from build123d import *
from build123d.topology import SkipClean

# Parameters (mm, degrees)
BOSS_EXTRUDE1_DEPTH   = 0.00254
BOSS_EXTRUDE1_2_DEPTH = 0.00254
BOSS_EXTRUDE1_3_DEPTH = 0.00254
BOSS_EXTRUDE1_4_DEPTH = 0.00254
SKETCH1_3_R           = 4.7625
BOSS_EXTRUDE2_DEPTH   = 1.9812
SKETCH1_6_R           = 14.02334
BOSS_EXTRUDE4_DEPTH   = 1.9812
SKETCH1_7_R           = 18.669
SKETCH1_7_R_2         = 14.02334
BOSS_EXTRUDE5_DEPTH   = 21.4122
BOSS_EXTRUDE6_DEPTH   = 21.4122
BOSS_EXTRUDE7_DEPTH   = 80.264
SKETCH9_R             = 4.064
CUT_EXTRUDE6_DEPTH    = 11.938
SKETCH10_R            = 3.556
CUT_EXTRUDE7_DEPTH    = 25.4


with BuildPart() as part:
    # Sketch1 → Boss-Extrude1 (new body)
    with BuildSketch(Plane.XY):
        with BuildLine():
            add(Edge.make_bspline(
                [(-11.267882352, 10.780839024), (-10.870534927, 8.031966006), (-8.087704817, 8.031966006), (-5.304874707, 8.031966006), (-4.907527282, 10.780839024)],
                knots=[3.284867705, 3.284867705, 3.284867705, 4.71238898, 4.71238898, 6.139910255, 6.139910255, 6.139910255], degree=2, weights=[1, 0.755905209, 1, 0.755905209, 1]))
            add(Edge.make_bspline(
                [(-4.907527282, 10.780839024), (-4.377808345, 14.445466006), (-8.087704817, 14.445466006), (-11.79760129, 14.445466006), (-11.267882352, 10.780839024)],
                knots=[6.139910255, 6.139910255, 6.139910255, 7.853981634, 7.853981634, 9.568053013, 9.568053013, 9.568053013], degree=2, weights=[1, 0.654681079, 1, 0.654681079, 1]))
        make_face()
    extrude(amount=BOSS_EXTRUDE1_DEPTH)



with BuildPart() as body_2:
    # Sketch1 → Boss-Extrude1 2 (new body)
    with BuildSketch(Plane.XY):
        with BuildLine():
            add(Edge.make_bspline(
                [(-15.980077835, -0.291711529), (-13.231204817, 0.105635896), (-13.231204817, 2.888466006), (-13.231204817, 5.671296116), (-15.980077835, 6.068643541)],
                knots=[3.284867705, 3.284867705, 3.284867705, 4.71238898, 4.71238898, 6.139910255, 6.139910255, 6.139910255], degree=2, weights=[1, 0.755905209, 1, 0.755905209, 1]))
            add(Edge.make_bspline(
                [(-15.980077835, 6.068643541), (-19.644704817, 6.598362479), (-19.644704817, 2.888466006), (-19.644704817, -0.821430466), (-15.980077835, -0.291711529)],
                knots=[6.139910255, 6.139910255, 6.139910255, 7.853981634, 7.853981634, 9.568053013, 9.568053013, 9.568053013], degree=2, weights=[1, 0.654681079, 1, 0.654681079, 1]))
        make_face()
    extrude(amount=BOSS_EXTRUDE1_2_DEPTH)


with BuildPart() as body_3:
    # Sketch1 → Boss-Extrude1 3 (new body)
    with BuildSketch(Plane.XY):
        with BuildLine():
            add(Edge.make_bspline(
                [(-4.907527282, -5.003907011), (-5.304874707, -2.255033994), (-8.087704817, -2.255033994), (-10.870534927, -2.255033994), (-11.267882352, -5.003907011)],
                knots=[3.284867705, 3.284867705, 3.284867705, 4.71238898, 4.71238898, 6.139910255, 6.139910255, 6.139910255], degree=2, weights=[1, 0.755905209, 1, 0.755905209, 1]))
            add(Edge.make_bspline(
                [(-11.267882352, -5.003907011), (-11.79760129, -8.668533994), (-8.087704817, -8.668533994), (-4.377808345, -8.668533994), (-4.907527282, -5.003907011)],
                knots=[6.139910255, 6.139910255, 6.139910255, 7.853981634, 7.853981634, 9.568053013, 9.568053013, 9.568053013], degree=2, weights=[1, 0.654681079, 1, 0.654681079, 1]))
        make_face()
    extrude(amount=BOSS_EXTRUDE1_3_DEPTH)


with BuildPart() as body_4:
    # Sketch1 → Boss-Extrude1 4 (new body)
    with BuildSketch(Plane.XY):
        with BuildLine():
            add(Edge.make_bspline(
                [(-0.1953318, 6.068643541), (-2.944204817, 5.671296116), (-2.944204817, 2.888466006), (-2.944204817, 0.105635896), (-0.1953318, -0.291711529)],
                knots=[3.284867705, 3.284867705, 3.284867705, 4.71238898, 4.71238898, 6.139910255, 6.139910255, 6.139910255], degree=2, weights=[1, 0.755905209, 1, 0.755905209, 1]))
            add(Edge.make_bspline(
                [(-0.1953318, -0.291711529), (3.469295183, -0.821430466), (3.469295183, 2.888466006), (3.469295183, 6.598362479), (-0.1953318, 6.068643541)],
                knots=[6.139910255, 6.139910255, 6.139910255, 7.853981634, 7.853981634, 9.568053013, 9.568053013, 9.568053013], degree=2, weights=[1, 0.654681079, 1, 0.654681079, 1]))
        make_face()
    extrude(amount=BOSS_EXTRUDE1_4_DEPTH)


with BuildPart() as part_1:
    add(part.part)

    add(body_2.part)  # Boss-Extrude2 merges body 2

    add(body_3.part)  # Boss-Extrude2 merges body 3

    add(body_4.part)  # Boss-Extrude2 merges body 4
    # Sketch1<3> → Boss-Extrude2 (add)
    with BuildSketch(Plane.XY):
        with BuildLine():
            ThreePointArc((-0.1953318, 6.068643541), (-2.070933216, 8.905237607), (-4.907527282, 10.780839024))
            add(Edge.make_bspline(
                [(-11.267882352, 10.780839024), (-10.870534927, 8.031966006), (-8.087704817, 8.031966006), (-5.304874707, 8.031966006), (-4.907527282, 10.780839024)],
                knots=[3.284867705, 3.284867705, 3.284867705, 4.71238898, 4.71238898, 6.139910255, 6.139910255, 6.139910255], degree=2, weights=[1, 0.755905209, 1, 0.755905209, 1]))
            ThreePointArc((-11.267882352, 10.780839024), (-14.104476418, 8.905237607), (-15.980077835, 6.068643541))
            add(Edge.make_bspline(
                [(-15.980077835, -0.291711529), (-13.231204817, 0.105635896), (-13.231204817, 2.888466006), (-13.231204817, 5.671296116), (-15.980077835, 6.068643541)],
                knots=[3.284867705, 3.284867705, 3.284867705, 4.71238898, 4.71238898, 6.139910255, 6.139910255, 6.139910255], degree=2, weights=[1, 0.755905209, 1, 0.755905209, 1]))
            ThreePointArc((-15.980077835, -0.291711529), (-14.104476418, -3.128305595), (-11.267882352, -5.003907011))
            add(Edge.make_bspline(
                [(-4.907527282, -5.003907011), (-5.304874707, -2.255033994), (-8.087704817, -2.255033994), (-10.870534927, -2.255033994), (-11.267882352, -5.003907011)],
                knots=[3.284867705, 3.284867705, 3.284867705, 4.71238898, 4.71238898, 6.139910255, 6.139910255, 6.139910255], degree=2, weights=[1, 0.755905209, 1, 0.755905209, 1]))
            ThreePointArc((-4.907527282, -5.003907011), (-2.070933216, -3.128305595), (-0.1953318, -0.291711529))
            add(Edge.make_bspline(
                [(-0.1953318, 6.068643541), (-2.944204817, 5.671296116), (-2.944204817, 2.888466006), (-2.944204817, 0.105635896), (-0.1953318, -0.291711529)],
                knots=[3.284867705, 3.284867705, 3.284867705, 4.71238898, 4.71238898, 6.139910255, 6.139910255, 6.139910255], degree=2, weights=[1, 0.755905209, 1, 0.755905209, 1]))
        make_face()
        with Locations((-8.087704817, 2.888466006)):
            Circle(SKETCH1_3_R, mode=Mode.SUBTRACT)
    extrude(amount=BOSS_EXTRUDE2_DEPTH)

    # Sketch1<6> → Boss-Extrude4 (add)
    with BuildSketch(Plane.XY):
        with Locations((-8.087704817, 2.888466006)):
            Circle(SKETCH1_6_R)
        with BuildLine():
            add(Edge.make_bspline(
                [(-15.980077835, 6.068643541), (-19.644704817, 6.598362479), (-19.644704817, 2.888466006), (-19.644704817, -0.821430466), (-15.980077835, -0.291711529)],
                knots=[6.139910255, 6.139910255, 6.139910255, 7.853981634, 7.853981634, 9.568053013, 9.568053013, 9.568053013], degree=2, weights=[1, 0.654681079, 1, 0.654681079, 1]))
            ThreePointArc((-15.980077835, -0.291711529), (-14.104476418, -3.128305595), (-11.267882352, -5.003907011))
            add(Edge.make_bspline(
                [(-11.267882352, -5.003907011), (-11.79760129, -8.668533994), (-8.087704817, -8.668533994), (-4.377808345, -8.668533994), (-4.907527282, -5.003907011)],
                knots=[6.139910255, 6.139910255, 6.139910255, 7.853981634, 7.853981634, 9.568053013, 9.568053013, 9.568053013], degree=2, weights=[1, 0.654681079, 1, 0.654681079, 1]))
            ThreePointArc((-4.907527282, -5.003907011), (-2.070933216, -3.128305595), (-0.1953318, -0.291711529))
            add(Edge.make_bspline(
                [(-0.1953318, -0.291711529), (3.469295183, -0.821430466), (3.469295183, 2.888466006), (3.469295183, 6.598362479), (-0.1953318, 6.068643541)],
                knots=[6.139910255, 6.139910255, 6.139910255, 7.853981634, 7.853981634, 9.568053013, 9.568053013, 9.568053013], degree=2, weights=[1, 0.654681079, 1, 0.654681079, 1]))
            ThreePointArc((-0.1953318, 6.068643541), (-2.070933216, 8.905237607), (-4.907527282, 10.780839024))
            add(Edge.make_bspline(
                [(-4.907527282, 10.780839024), (-4.377808345, 14.445466006), (-8.087704817, 14.445466006), (-11.79760129, 14.445466006), (-11.267882352, 10.780839024)],
                knots=[6.139910255, 6.139910255, 6.139910255, 7.853981634, 7.853981634, 9.568053013, 9.568053013, 9.568053013], degree=2, weights=[1, 0.654681079, 1, 0.654681079, 1]))
            ThreePointArc((-11.267882352, 10.780839024), (-14.104476418, 8.905237607), (-15.980077835, 6.068643541))
        make_face(mode=Mode.SUBTRACT)
    extrude(amount=BOSS_EXTRUDE4_DEPTH)

    # Sketch1<7> → Boss-Extrude5 (add)
    with BuildSketch(Plane.XY):
        with Locations((-8.087704817, 2.888466006)):
            Circle(SKETCH1_7_R)
        with Locations((-8.087704817, 2.888466006)):
            Circle(SKETCH1_7_R_2, mode=Mode.SUBTRACT)
    extrude(amount=BOSS_EXTRUDE5_DEPTH)

    # Sketch2 → Boss-Extrude6 (add, through all)
    with BuildSketch(Plane.XY.offset(21.4122)):
        with BuildLine():
            ThreePointArc((-16.011919536, 19.792263866), (-7.867306443, 21.556164995), (0.233391542, 19.60046518))
            ThreePointArc((0.233391542, 19.60046518), (-0.607958843, 22.777981932), (0.25217674, 25.95046518))
            Line((0.25217674, 25.95046518), (-16.25782326, 25.95046518))
            ThreePointArc((-16.25782326, 25.95046518), (-15.337670431, 22.903197631), (-16.011919536, 19.792263866))
        make_face()
        with BuildLine():
            ThreePointArc((0.233391542, -13.823533167), (-7.867306443, -15.779232983), (-16.011919536, -14.015331854))
            ThreePointArc((-16.011919536, -14.015331854), (-15.337670431, -17.126265618), (-16.25782326, -20.173533167))
            Line((-16.25782326, -20.173533167), (0.25217674, -20.173533167))
            ThreePointArc((0.25217674, -20.173533167), (-0.607958843, -17.001049919), (0.233391542, -13.823533167))
        make_face()
    extrude(amount=-BOSS_EXTRUDE6_DEPTH)

    # Sketch3 → Boss-Extrude7 (add)
    with SkipClean():  # the faces are left unmerged after this step: merging them gives an invalid solid
        with BuildSketch(Plane(origin=(0, 0, 0), x_dir=(-1, 0, 0), z_dir=(0, 0, -1))):
            with BuildLine():
                ThreePointArc((16.011919536, 19.792263866), (15.337670431, 22.903197631), (16.25782326, 25.95046518))
                Line((16.25782326, 25.95046518), (-0.25217674, 25.95046518))
                ThreePointArc((-0.25217674, 25.95046518), (0.607958843, 22.777981932), (-0.233391542, 19.60046518))
                ThreePointArc((-0.233391542, 19.60046518), (-10.581295183, 2.888466006), (-0.233391542, -13.823533167))
                ThreePointArc((-0.233391542, -13.823533167), (0.607958843, -17.001049919), (-0.25217674, -20.173533167))
                Line((-0.25217674, -20.173533167), (16.25782326, -20.173533167))
                ThreePointArc((16.25782326, -20.173533167), (15.337670431, -17.126265618), (16.011919536, -14.015331854))
                ThreePointArc((16.011919536, -14.015331854), (26.756704817, 2.888466006), (16.011919536, 19.792263866))
            make_face()
        extrude(amount=BOSS_EXTRUDE7_DEPTH)

    # Sketch9 → Cut-Extrude6 (cut)
    with SkipClean():  # the faces are left unmerged after this step: merging them gives an invalid solid
        with BuildSketch(Plane.XY):
            with Locations((-8.087704817, 2.888466006)):
                Circle(SKETCH9_R)
        extrude(amount=-CUT_EXTRUDE6_DEPTH, mode=Mode.SUBTRACT)

    # Sketch10 → Cut-Extrude7 (cut)
    with SkipClean():  # the faces are left unmerged after this step: merging them gives an invalid solid
        with BuildSketch(Plane(origin=(0, 0, -80.264), x_dir=(-1, 0, 0), z_dir=(0, 0, -1))):
            with Locations((8.087704817, 2.888466006)):
                Circle(SKETCH10_R)
        extrude(amount=-CUT_EXTRUDE7_DEPTH, mode=Mode.SUBTRACT)


solid = part_1.part
The model under review builds one solid part; all positions refer to its coordinate system, in mm. A direction names the side the tool comes from. Give positions to 0.01 mm unless a question says otherwise; leave off trailing zeros. Loops run counter-clockwise (first coordinate to the right, second up) from the corner with the lowest first, then second, coordinate; pieces in that order, holes last. Notation, with made-up numbers: (-3.75, -30) -> (44.25, -30) arc R28 cw to (44.25, 6) -> close; hole circle Ø8 at (22.25, 17.25). An arc over 180 degrees is marked (long way). Answer as a JSON object with one key per item and string values. Group by question number.
Q1. Wall thickness on line 1 along X through (y, z) = (3, -74.5); line 2 along Z through (x, y) = (-19.5, -3); line 3 along Y through (x, z) = (2.5, 15.5): over which ranges is each line inside the solid? List them lowest first.
Q2. Take a section at B-B (z = -73). Write out the cut boundary in (x, y), plus the area to 3 significant figures.
Q3. Take a section at A-A (z = -16). Write out the cut boundary in (x, y).
Q4. Take a section at C-C (y = -16.5). Write out the cut boundary in (x, z).
Q5. Draft analysis for pull direction X (two halves, no side actions). For faces 4 (the flat face through (-4, -11, 21.412)), 5 (the cylindrical face through (-8.97, -1.08, -5.89)), 6 (the cylindrical face through (-0.608, 22.825, -28.714)), 7 (the flat face through (-16, 3, 0.003)), state which applies: pulls with the +X half, pulls with the -X half, needs draft (parallel to the pull), parting line crosses it, or undercut.
Q6. Tool access review of faces 1 (the flat face through (-8, 3, -54.864)), 2 (the flat face through (-12, 5, 0)), 3 (the flat face through (-8, -20.174, -29)): name each direction out of +Z, -Z, +X, -X, +Y, -Y from which nothing blocks a thin tool from reaching the whole face with its end or side.
Q7. Insertion check: pin 1 (7 mm diameter, centred on x = 1.5, y = 4, fed in from +Z); pin 2 (5.5 mm diameter, centred on x = -6.5, y = 2.5, fed in from -Z); pin 3 (10 mm diameter, centred on y = 17, z = -20.5, fed in from +X); pin 4 (2.5 mm diameter, centred on x = -6.5, y = 1, fed in from +Z). Each pin has a flat end and moves straight along its axis. Give the tip position at first contact, or say it passes through.
Q8. Take a section at D-D (y = 21). Write out the cut boundary in (x, z), plus the area to 3 significant figures.
Answer below:
{
 "1": {"line 1": "x = -26.76 to -11.64, -4.53 to 10.58", "line 2": "z = -80.26 to 1.98", "line 3": "y = -12.49 to -6.31, 12.08 to 18.26"},
 "2": {"outline": "(-16.26, -20.17) -> (0.25, -20.17) arc R6.35 cw to (0.23, -13.82) arc R18.67 ccw to (0.23, 19.6) arc R6.35 cw to (0.25, 25.95) -> (-16.26, 25.95) arc R6.35 cw to (-16.01, 19.79) arc R18.67 ccw to (-16.01, -14.02) arc R6.35 cw to start; hole circle Ø7.11 at (-8.09, 2.89)", "area": "1,210 mm2"},
 "3": {"outline": "(-16.26, -20.17) -> (0.25, -20.17) arc R6.35 cw to (0.23, -13.82) arc R18.67 ccw to (0.23, 19.6) arc R6.35 cw to (0.25, 25.95) -> (-16.26, 25.95) arc R6.35 cw to (-16.01, 19.79) arc R18.67 ccw to (-16.01, -14.02) arc R6.35 cw to start"},
 "4": {"outline": "(-15.34, -80.26) -> (-0.59, -80.26) -> (-0.59, 21.41) -> (-15.34, 21.41) -> close"},
 "5": {"face 4": "needs draft", "face 5": "undercut", "face 6": "pulls with the +X half", "face 7": "undercut"},
 "6": {"face 1": "-Z", "face 2": "+Z", "face 3": "+Z, -Z, +X, -X, -Y"},
 "7": {"pin 1": "stops at z = 1.98", "pin 2": "stops at z = -80.26", "pin 3": "stops at x = 8.21", "pin 4": "stops at z = -11.94"},
 "8": {"outline": "(-15.55, -80.26) -> (-0.36, -80.26) -> (-0.36, 21.41) -> (-15.55, 21.41) -> close", "area": "1,540 mm2"}
}
